Check sheet for the modelled part. Datum: model origin and axes. Units: mm. A direction names the side the tool comes from. Round coordinates to 2 decimals unless told otherwise and drop trailing zeros. Loops run counter-clockwise (first coordinate to the right, second up) from the corner with the lowest first, then second, coordinate; pieces in that order, holes last. Notation, with made-up numbers: (86, 13.5) - (128, 13.5) arc R20 ccw to (128, 25.5) - close; hole circle Ø5 at (49, 13). An arc over 180 degrees is marked (long way). Return JSON: item names as keys, results as strings.
from build123d import *

# Parameters (mm, degrees)
SKETCH1_W            = 80
SKETCH1_H            = 130
BOSS_EXTRUDE1_DEPTH  = 10
BOSS_EXTRUDE10_DEPTH = 42.3
SKETCH13_W           = 115
SKETCH13_H           = 39.8
CUT_EXTRUDE3_DEPTH   = 11
SKETCH14_W           = 65
SKETCH14_H           = 39.8
CUT_EXTRUDE4_DEPTH   = 11
SKETCH15_R           = 1.5
CUT_EXTRUDE5_DEPTH   = 4
SKETCH21_R           = 2.1
CUT_EXTRUDE8_DEPTH   = 11
BOSS_EXTRUDE11_DEPTH = 5
CUT_EXTRUDE9_DEPTH   = 11
SKETCH24_R           = 1.5
CUT_EXTRUDE10_DEPTH  = 4
SKETCH25_W           = 12.5
SKETCH25_H           = 8
CUT_EXTRUDE11_DEPTH  = 6


with BuildPart() as part:
    # Sketch1 → Boss-Extrude1 (new body)
    with BuildSketch(Plane(origin=(0, 0, 0), x_dir=(1, 0, 0), z_dir=(0, 1, 0))):
        with Locations((-5, 5)):
            Rectangle(SKETCH1_W, SKETCH1_H)
    extrude(amount=BOSS_EXTRUDE1_DEPTH)

    # Sketch9 → Boss-Extrude10 (add)
    with BuildSketch(Plane(origin=(0, 10, 0), x_dir=(1, 0, 0), z_dir=(0, 1, 0))):
        Polygon((35, 70), (-45, 70), (-45, -60), (-35, -60), (-35, 60), (35, 60), align=None)
    extrude(amount=BOSS_EXTRUDE10_DEPTH)

    # Sketch13 → Cut-Extrude3 (cut, through all)
    with BuildSketch(Plane(origin=(-35, 0, 0), x_dir=(0, 0, -1), z_dir=(1, 0, 0))):
        with Locations((2.5, 32.4)):
            Rectangle(SKETCH13_W, SKETCH13_H)
    extrude(amount=-CUT_EXTRUDE3_DEPTH, mode=Mode.SUBTRACT)

    # Sketch14 → Cut-Extrude4 (cut, through all)
    with BuildSketch(Plane.XY.offset(-60)):
        with Locations((-2.5, 32.4)):
            Rectangle(SKETCH14_W, SKETCH14_H)
    extrude(amount=-CUT_EXTRUDE4_DEPTH, mode=Mode.SUBTRACT)

    # Sketch15 → Cut-Extrude5 (cut)
    with BuildSketch(Plane(origin=(0, 52.3, 0), x_dir=(1, 0, 0), z_dir=(0, 1, 0))):
        with Locations((-40, 65)):
            Circle(SKETCH15_R)
    extrude(amount=-CUT_EXTRUDE5_DEPTH, mode=Mode.SUBTRACT)

    # Sketch21 → Cut-Extrude8 (cut, through all)
    with BuildSketch(Plane(origin=(0, 10, 0), x_dir=(1, 0, 0), z_dir=(0, 1, 0))):
        with Locations((-26.5, 42)):
            Circle(SKETCH21_R)
    extrude(amount=-CUT_EXTRUDE8_DEPTH, mode=Mode.SUBTRACT)

    # Sketch22 → Boss-Extrude11 (add)
    with BuildSketch(Plane(origin=(35, 0, 0), x_dir=(0, 0, -1), z_dir=(1, 0, 0))):
        with BuildLine():
            Line((-0.212132034, 8.037867966), (-3.037867966, 5.212132034))
            ThreePointArc((-3.037867966, 5.212132034), (-3.125735931, 5), (-3.037867966, 4.787867966))
            Line((-3.037867966, 4.787867966), (-0.212132034, 1.962132034))
            ThreePointArc((-0.212132034, 1.962132034), (0, 1.874264069), (0.212132034, 1.962132034))
            Line((0.212132034, 1.962132034), (3.037867966, 4.787867966))
            ThreePointArc((3.037867966, 4.787867966), (3.125735931, 5), (3.037867966, 5.212132034))
            Line((3.037867966, 5.212132034), (0.212132034, 8.037867966))
            ThreePointArc((0.212132034, 8.037867966), (0, 8.125735931), (-0.212132034, 8.037867966))
        make_face()
        with BuildLine():
            Line((15.537867966, 5.212132034), (12.712132034, 8.037867966))
            ThreePointArc((12.712132034, 8.037867966), (12.5, 8.125735931), (12.287867966, 8.037867966))
            Line((12.287867966, 8.037867966), (9.462132034, 5.212132034))
            ThreePointArc((9.462132034, 5.212132034), (9.374264069, 5), (9.462132034, 4.787867966))
            Line((9.462132034, 4.787867966), (12.287867966, 1.962132034))
            ThreePointArc((12.287867966, 1.962132034), (12.5, 1.874264069), (12.712132034, 1.962132034))
            Line((12.712132034, 1.962132034), (15.537867966, 4.787867966))
            ThreePointArc((15.537867966, 4.787867966), (15.625735931, 5), (15.537867966, 5.212132034))
        make_face()
        with BuildLine():
            Line((28.037867966, 5.212132034), (25.212132034, 8.037867966))
            ThreePointArc((25.212132034, 8.037867966), (25, 8.125735931), (24.787867966, 8.037867966))
            Line((24.787867966, 8.037867966), (21.962132034, 5.212132034))
            ThreePointArc((21.962132034, 5.212132034), (21.874264069, 5), (21.962132034, 4.787867966))
            Line((21.962132034, 4.787867966), (24.787867966, 1.962132034))
            ThreePointArc((24.787867966, 1.962132034), (25, 1.874264069), (25.212132034, 1.962132034))
            Line((25.212132034, 1.962132034), (28.037867966, 4.787867966))
            ThreePointArc((28.037867966, 4.787867966), (28.125735931, 5), (28.037867966, 5.212132034))
        make_face()
        with BuildLine():
            Line((40.537867966, 5.212132034), (37.712132034, 8.037867966))
            ThreePointArc((37.712132034, 8.037867966), (37.5, 8.125735931), (37.287867966, 8.037867966))
            Line((37.287867966, 8.037867966), (34.462132034, 5.212132034))
            ThreePointArc((34.462132034, 5.212132034), (34.374264069, 5), (34.462132034, 4.787867966))
            Line((34.462132034, 4.787867966), (37.287867966, 1.962132034))
            ThreePointArc((37.287867966, 1.962132034), (37.5, 1.874264069), (37.712132034, 1.962132034))
            Line((37.712132034, 1.962132034), (40.537867966, 4.787867966))
            ThreePointArc((40.537867966, 4.787867966), (40.625735931, 5), (40.537867966, 5.212132034))
        make_face()
        with BuildLine():
            Line((53.037867966, 5.212132034), (50.212132034, 8.037867966))
            ThreePointArc((50.212132034, 8.037867966), (50, 8.125735931), (49.787867966, 8.037867966))
            Line((49.787867966, 8.037867966), (46.962132034, 5.212132034))
            ThreePointArc((46.962132034, 5.212132034), (46.874264069, 5), (46.962132034, 4.787867966))
            Line((46.962132034, 4.787867966), (49.787867966, 1.962132034))
            ThreePointArc((49.787867966, 1.962132034), (50, 1.874264069), (50.212132034, 1.962132034))
            Line((50.212132034, 1.962132034), (53.037867966, 4.787867966))
            ThreePointArc((53.037867966, 4.787867966), (53.125735931, 5), (53.037867966, 5.212132034))
        make_face()
        with BuildLine():
            Line((65.537867966, 5.212132034), (62.712132034, 8.037867966))
            ThreePointArc((62.712132034, 8.037867966), (62.5, 8.125735931), (62.287867966, 8.037867966))
            Line((62.287867966, 8.037867966), (59.462132034, 5.212132034))
            ThreePointArc((59.462132034, 5.212132034), (59.374264069, 5), (59.462132034, 4.787867966))
            Line((59.462132034, 4.787867966), (62.287867966, 1.962132034))
            ThreePointArc((62.287867966, 1.962132034), (62.5, 1.874264069), (62.712132034, 1.962132034))
            Line((62.712132034, 1.962132034), (65.537867966, 4.787867966))
            ThreePointArc((65.537867966, 4.787867966), (65.625735931, 5), (65.537867966, 5.212132034))
        make_face()
        with BuildLine():
            Line((-9.462132034, 5.212132034), (-12.287867966, 8.037867966))
            ThreePointArc((-12.287867966, 8.037867966), (-12.5, 8.125735931), (-12.712132034, 8.037867966))
            Line((-12.712132034, 8.037867966), (-15.537867966, 5.212132034))
            ThreePointArc((-15.537867966, 5.212132034), (-15.625735931, 5), (-15.537867966, 4.787867966))
            Line((-15.537867966, 4.787867966), (-12.712132034, 1.962132034))
            ThreePointArc((-12.712132034, 1.962132034), (-12.5, 1.874264069), (-12.287867966, 1.962132034))
            Line((-12.287867966, 1.962132034), (-9.462132034, 4.787867966))
            ThreePointArc((-9.462132034, 4.787867966), (-9.374264069, 5), (-9.462132034, 5.212132034))
        make_face()
        with BuildLine():
            Line((-21.962132034, 5.212132034), (-24.787867966, 8.037867966))
            ThreePointArc((-24.787867966, 8.037867966), (-25, 8.125735931), (-25.212132034, 8.037867966))
            Line((-25.212132034, 8.037867966), (-28.037867966, 5.212132034))
            ThreePointArc((-28.037867966, 5.212132034), (-28.125735931, 5), (-28.037867966, 4.787867966))
            Line((-28.037867966, 4.787867966), (-25.212132034, 1.962132034))
            ThreePointArc((-25.212132034, 1.962132034), (-25, 1.874264069), (-24.787867966, 1.962132034))
            Line((-24.787867966, 1.962132034), (-21.962132034, 4.787867966))
            ThreePointArc((-21.962132034, 4.787867966), (-21.874264069, 5), (-21.962132034, 5.212132034))
        make_face()
        with BuildLine():
            Line((-34.462132034, 5.212132034), (-37.287867966, 8.037867966))
            ThreePointArc((-37.287867966, 8.037867966), (-37.5, 8.125735931), (-37.712132034, 8.037867966))
            Line((-37.712132034, 8.037867966), (-40.537867966, 5.212132034))
            ThreePointArc((-40.537867966, 5.212132034), (-40.625735931, 5), (-40.537867966, 4.787867966))
            Line((-40.537867966, 4.787867966), (-37.712132034, 1.962132034))
            ThreePointArc((-37.712132034, 1.962132034), (-37.5, 1.874264069), (-37.287867966, 1.962132034))
            Line((-37.287867966, 1.962132034), (-34.462132034, 4.787867966))
            ThreePointArc((-34.462132034, 4.787867966), (-34.374264069, 5), (-34.462132034, 5.212132034))
        make_face()
        with BuildLine():
            Line((-46.962132034, 5.212132034), (-49.787867966, 8.037867966))
            ThreePointArc((-49.787867966, 8.037867966), (-50, 8.125735931), (-50.212132034, 8.037867966))
            Line((-50.212132034, 8.037867966), (-53.037867966, 5.212132034))
            ThreePointArc((-53.037867966, 5.212132034), (-53.125735931, 5), (-53.037867966, 4.787867966))
            Line((-53.037867966, 4.787867966), (-50.212132034, 1.962132034))
            ThreePointArc((-50.212132034, 1.962132034), (-50, 1.874264069), (-49.787867966, 1.962132034))
            Line((-49.787867966, 1.962132034), (-46.962132034, 4.787867966))
            ThreePointArc((-46.962132034, 4.787867966), (-46.874264069, 5), (-46.962132034, 5.212132034))
        make_face()
        with BuildLine():
            Line((61.962132034, 31.362132034), (64.787867966, 34.187867966))
            ThreePointArc((64.787867966, 34.187867966), (65, 34.275735931), (65.212132034, 34.187867966))
            Line((65.212132034, 34.187867966), (68.037867966, 31.362132034))
            ThreePointArc((68.037867966, 31.362132034), (68.125735931, 31.15), (68.037867966, 30.937867966))
            Line((68.037867966, 30.937867966), (65.212132034, 28.112132034))
            ThreePointArc((65.212132034, 28.112132034), (65, 28.024264069), (64.787867966, 28.112132034))
            Line((64.787867966, 28.112132034), (61.962132034, 30.937867966))
            ThreePointArc((61.962132034, 30.937867966), (61.874264069, 31.15), (61.962132034, 31.362132034))
        make_face()
        with BuildLine():
            Line((64.787867966, 40.612132034), (61.962132034, 43.437867966))
            ThreePointArc((61.962132034, 43.437867966), (61.874264069, 43.65), (61.962132034, 43.862132034))
            Line((61.962132034, 43.862132034), (64.787867966, 46.687867966))
            ThreePointArc((64.787867966, 46.687867966), (65, 46.775735931), (65.212132034, 46.687867966))
            Line((65.212132034, 46.687867966), (68.037867966, 43.862132034))
            ThreePointArc((68.037867966, 43.862132034), (68.125735931, 43.65), (68.037867966, 43.437867966))
            Line((68.037867966, 43.437867966), (65.212132034, 40.612132034))
            ThreePointArc((65.212132034, 40.612132034), (65, 40.524264069), (64.787867966, 40.612132034))
        make_face()
        with BuildLine():
            Line((64.787867966, 15.612132034), (61.962132034, 18.437867966))
            ThreePointArc((61.962132034, 18.437867966), (61.874264069, 18.65), (61.962132034, 18.862132034))
            Line((61.962132034, 18.862132034), (64.787867966, 21.687867966))
            ThreePointArc((64.787867966, 21.687867966), (65, 21.775735931), (65.212132034, 21.687867966))
            Line((65.212132034, 21.687867966), (68.037867966, 18.862132034))
            ThreePointArc((68.037867966, 18.862132034), (68.125735931, 18.65), (68.037867966, 18.437867966))
            Line((68.037867966, 18.437867966), (65.212132034, 15.612132034))
            ThreePointArc((65.212132034, 15.612132034), (65, 15.524264069), (64.787867966, 15.612132034))
        make_face()
    extrude(amount=BOSS_EXTRUDE11_DEPTH)

    # Sketch23 → Cut-Extrude9 (cut, through all)
    with BuildSketch(Plane(origin=(0, 10, 0), x_dir=(1, 0, 0), z_dir=(0, 1, 0))):
        Polygon((30, -55), (-35, -55), (-35, 38), (-22.5, 38), (-22.5, 46), (-35, 46), (-35, 60), (30, 60), align=None)
    extrude(amount=-CUT_EXTRUDE9_DEPTH, mode=Mode.SUBTRACT)

    # Sketch24 → Cut-Extrude10 (cut)
    with BuildSketch(Plane.XZ):
        with Locations((-40, -65)):
            Circle(SKETCH24_R)
    extrude(amount=-CUT_EXTRUDE10_DEPTH, mode=Mode.SUBTRACT)

    # Sketch25 → Cut-Extrude11 (cut)
    with BuildSketch(Plane.XZ):
        with Locations((-28.75, -42)):
            Rectangle(SKETCH25_W, SKETCH25_H)
    extrude(amount=-CUT_EXTRUDE11_DEPTH, mode=Mode.SUBTRACT)


solid = part.part
Q1. Draft check along Y on faces 1 (the face through (37.5, 32.8, -66.6)), 2 (the face through (37.47, 6.64, 51.61)), 3 (the face through (40, 5, -50)), 4 (the face through (37.47, 3.36, 23.39)). Enter one of: released by +Y, released by -Y, zero draft, split by the parting line, or undercut.
Answer key:
{"face 1": "undercut", "face 2": "released by +Y", "face 3": "zero draft", "face 4": "released by -Y"}
Q2. Sectioned sample at B-B (y = 24). Enter the section's corners in (x, z), plus the area to 3 significant figures.
Answer key:
{"outline": "(-45, -70) - (-35, -70) - (-35, -60) - (-45, -60) - close; (-45, 55) - (-35, 55) - (-35, 60) - (-45, 60) - close; (30, -70) - (35, -70) - (35, -60) - (30, -60) - close", "area": "200 mm²"}
Q3. Tool access check on faces 5 (the face through (-40, 48.3, -65)), 6 (the face through (37.47, 3.36, -64.11)), 7 (the face through (37.47, 3.39, -48.36)), 8 (the face through (37.47, 6.61, 35.86)), 9 (the face through (-35, 32, -65)). Record the directions out of +Z, -Z, +X, -X, +Y, -Y that give a thin tool (end or side, any length) a straight path to the whole face; none if there is none.
Answer key:
{"face 5": "+Y", "face 6": "-Z, +X, -Y", "face 7": "+X, -Y", "face 8": "+X, +Y", "face 9": "+Z, -Z, +Y"}
Q4. Sectioned sample at A-A (z = -42). Enter the section's corners in (x, y).
Answer key:
{"outline": "(-45, 0) - (-35, 0) - (-35, 6) - (-28.6, 6) - (-28.6, 10) - (-35, 10) - (-35, 12.5) - (-45, 12.5) - close; (-24.4, 6) - (-22.5, 6) - (-22.5, 10) - (-24.4, 10) - close; (30, 0) - (35, 0) - (35, 10) - (30, 10) - close"}
Q5. Scan lines: probe 1 along Z at (x, y) = (-26.5, 7.85); probe 2 along Z at (x, y) = (-40, 51.5); probe 3 along X at (y, z) = (8, -42). Record each from-to range of solid material in increasing order. Write a range as [from, to].
Answer key:
{"probe 1": "z = [-70, -60], [-46, -44.1], [-39.9, -38], [55, 60]", "probe 2": "z = [-70, -66.5], [-63.5, -60], [55, 60]", "probe 3": "x = [-45, -28.6], [-24.4, -22.5], [30, 35]"}
Q6. Sectioned sample at D-D (z = 44). Enter the section's corners in (x, y), plus the area to 3 significant figures.
Answer key:
{"outline": "(-45, 0) - (-35, 0) - (-35, 12.5) - (-45, 12.5) - close; (30, 0) - (35, 0) - (35, 10) - (30, 10) - close", "area": "175 mm²"}
Q7. Depth check by flat-ended pin: P1, Ø5, axis at x = -39, z = -2, coming from the +Y side; P2, Ø2.5, axis at x = -40.5, z = -64.5, coming from the -Y side; P3, Ø6.5, axis at x = -28.5, z = -42, coming from the +Y side; P4, Ø4, axis at x = -31, z = -40.5, coming from the -Y side. Enter the tip coordinate at first touch or a pass-through.
Answer key:
{"P1": "stops at y = 12.5", "P2": "stops at y = 0", "P3": "stops at y = 10", "P4": "stops at y = 6"}
Q8. Sectioned sample at C-C (x = -16). Enter the section's corners in (y, z).
Answer key:
{"outline": "(0, -70) - (12.5, -70) - (12.5, -60) - (0, -60) - close; (0, 55) - (10, 55) - (10, 60) - (0, 60) - close"}
